```python
from build123d import *

# Parameters (mm, degrees)
ESQUISSE1_W             = 18
ESQUISSE1_H             = 20
ESQUISSE4_W             = 2.25
ESQUISSE4_H             = 5.1
ENL_V_MAT_EXTRU_1_DEPTH = 15
ESQUISSE6_W             = 1.45
ESQUISSE6_H             = 22.75


# Read off the part's stored shape, not the designer's step: Diamètre du perçage Ø4.0 (4)1
with BuildPart() as part:
    # Esquisse1 → Révolution1 (revolve)
    with BuildSketch(Plane.XY, mode=Mode.PRIVATE) as r_volution1_sk:
        with Locations((9, 12.75)):
            Rectangle(ESQUISSE1_W, ESQUISSE1_H)
    revolve(r_volution1_sk.sketch.rotate(Axis((0, 0, 0), (1, 0, 0)), 90), axis=Axis((0, 0, 0), (1, 0, 0)))

    # Diamètre du perçage Ø4.0 (4)1 outline → Diamètre du perçage Ø4.0 (4)1 (revolve, cut)
    with BuildSketch(Plane(origin=(0, -9.510565163, -3.090169944), x_dir=(0, 1, 0), z_dir=(0, 0, -1))):
        Polygon((0, 18), (0, 8.298278762), (2, 9.5), (2, 18), align=None)
    revolve(axis=Axis((0, -9.510565163, -3.090169944), (1, 0, 0)), mode=Mode.SUBTRACT)

    # Diam_tre du per_age _4.0 _4_1 2 outline → Diam_tre du per_age _4.0 _4_1 2 (revolve, cut)
    with BuildSketch(Plane(origin=(0, -5.877852523, 8.090169944), x_dir=(0, 1, 0), z_dir=(0, 0, -1))):
        Polygon((0, 18), (0, 8.298278762), (2, 9.5), (2, 18), align=None)
    revolve(axis=Axis((0, -5.877852523, 8.090169944), (1, 0, 0)), mode=Mode.SUBTRACT)

    # Diam_tre du per_age _4.0 _4_1 3 outline → Diam_tre du per_age _4.0 _4_1 3 (revolve, cut)
    with BuildSketch(Plane(origin=(0, 5.877852523, 8.090169944), x_dir=(0, 1, 0), z_dir=(0, 0, -1))):
        Polygon((0, 18), (0, 8.298278762), (2, 9.5), (2, 18), align=None)
    revolve(axis=Axis((0, 5.877852523, 8.090169944), (1, 0, 0)), mode=Mode.SUBTRACT)

    # Diam_tre du per_age _4.0 _4_1 4 outline → Diam_tre du per_age _4.0 _4_1 4 (revolve, cut)
    with BuildSketch(Plane(origin=(0, 9.510565163, -3.090169944), x_dir=(0, 1, 0), z_dir=(0, 0, -1))):
        Polygon((0, 18), (0, 8.298278762), (2, 9.5), (2, 18), align=None)
    revolve(axis=Axis((0, 9.510565163, -3.090169944), (1, 0, 0)), mode=Mode.SUBTRACT)

    # Diam_tre du per_age _4.0 _4_1 5 outline → Diam_tre du per_age _4.0 _4_1 5 (revolve, cut)
    with BuildSketch(Plane.YX.offset(10)):
        Polygon((0, 18), (0, 8.298278762), (2, 9.5), (2, 18), align=None)
    revolve(axis=Axis((0, 0, -10), (1, 0, 0)), mode=Mode.SUBTRACT)

    # Esquisse4 → Enlèv. mat.-Extru.1 (cut)
    with BuildSketch(Plane(origin=(18, 0, 0), x_dir=(0, 0, -1), z_dir=(1, 0, 0))):
        with Locations((-16.125, 0)):
            Rectangle(ESQUISSE4_W, ESQUISSE4_H)
    extrude(amount=-ENL_V_MAT_EXTRU_1_DEPTH, mode=Mode.SUBTRACT)

    # Esquisse6 → Dégagement M2.51 (revolve, cut)
    with BuildSketch(Plane.YZ.offset(9)):
        with Locations((0.725, 11.375)):
            Rectangle(ESQUISSE6_W, ESQUISSE6_H)
    revolve(axis=Axis((9, 0, -6.35), (0, 0, 1)), mode=Mode.SUBTRACT)


solid = part.part
```
CAD build for the part. Positions are in the model's coordinates, mm. A direction names the side the tool comes from. Round coordinates to 2 decimals unless told otherwise and drop trailing zeros. Loops run counter-clockwise (first coordinate to the right, second up) from the corner with the lowest first, then second, coordinate; pieces in that order, holes last. Notation, with made-up numbers: M -25.5,-7.5 L 5.5,-7.5 A19 ccw 5.5,25.5 Z; hole C 81.25,31.25 d6. An arc over 180 degrees is marked long. Return JSON: item names as keys, results as strings. Group by question number.
(1) Mould opens along Z. For faces 3 (the conical face through (8.51, -9.86, -3.07)), 4 (the cylindrical face through (9.13, -6.83, 21.7)), 5 (the cylindrical face through (10.416, -0.314, 8.757)) say: +Z half, -Z half, draft (parallel to the pull), parting line (faces both ways), or undercut.
(2) Wall check: probe 1 along Y at (x, z) = (13, 0); probe 2 along Y at (x, z) = (10, 6.5); probe 3 along Y at (x, z) = (9, 6.5). Give the ranges that are in metal, low to high. Write a range as [from, to].
(3) Saw through at A-A, the plane z = 0. List the corners of the cut face in (x, y), and give its area (3 significant figures).
(4) Tool access for faces 1 (the cylindrical face through (13.81, 5.44, 6.14)), 2 (the flat face through (18, 5, 0)): list every direction of +Z, -Z, +X, -X, +Y, -Y with a clear straight run to the whole face (end or side of a thin tool).
(5) Drop flat-ended pins along their axis: P1, Ø1.1, axis at x = 7.5, z = 15.5, coming from the -Y side; P2, Ø2.5, axis at y = -5.88, z = 8.09, coming from the +X side; P3, Ø10, axis at x = 12, z = -7.5, coming from the -Y side. Give the stop position or say it passes through.
(6) Saw through at C-C, the plane z = 11. List the corners of the cut face in (x, y), and give its area (3 significant figures).
(7) Saw through at B-B, the plane x = 4. List the corners of the cut face in (y, z), and give its area (3 significant figures).
(8) Saw through at D-D, the plane x = 12. List the corners of the cut face in (y, z).
Answer list:
{
 "1": {"face 3": "undercut", "face 4": "parting line", "face 5": "draft"},
 "2": {"probe 1": "[-22.75, -2.75], [2.75, 22.75]", "probe 2": "[-21.8, -7.09], [-4.66, -1.05], [1.05, 4.66], [7.09, 21.8]", "probe 3": "[-21.8, -1.45], [1.45, 21.8]"},
 "3": {"outline": "M 0,-22.75 L 18,-22.75 L 18,-2.75 L 0,-2.75 Z; M 0,2.75 L 18,2.75 L 18,22.75 L 0,22.75 Z", "area": "720 mm2"},
 "4": {"face 1": "+X", "face 2": "+Z, -Z, +X, +Y, -Y"},
 "5": {"P1": "y = -17.15", "P2": "x = 9.05", "P3": "y = -22.61"},
 "6": {"outline": "M 0,-19.91 L 18,-19.91 L 18,19.91 L 0,19.91 Z; hole C 9,0 d2.9", "area": "710 mm2"},
 "7": {"outline": "C 0,0 d45.5; hole C 0,0 d5.5; hole M -2.55,15 L 2.55,15 L 2.55,17.25 L -2.55,17.25 Z", "area": "1,590 mm2"},
 "8": {"outline": "C 0,0 d45.5; hole C -9.51,-3.09 d4; hole C -5.88,8.09 d4; hole C 0,0 d5.5; hole M -2.55,15 L 2.55,15 L 2.55,17.25 L -2.55,17.25 Z; hole C 0,-10 d4; hole C 5.88,8.09 d4; hole C 9.51,-3.09 d4"}
}
